Design review of the part built by this model. Coordinates are the model's own, in mm. A direction names the side the tool comes from. Give positions to 0.01 mm unless a question says otherwise; leave off trailing zeros. Order: outer loops, then holes, each group sorted by start corner. A loop starts at its lowest first (then second) coordinate and runs counter-clockwise, first axis right, second up. Notation, with made-up numbers: (80.25, 1.25) -> (131.25, 1.25) arc R11 ccw to (131.25, 10.25) -> close; hole circle Ø4 at (-26.5, -29.5). An arc over 180 degrees is marked (long way). One line per item, written item: value.
from build123d import *

# Parameters (mm, degrees)
SKETCH_1_R          = 40
EXTRUDE_1_DEPTH     = 30
CUT_EXTRUDE_1_DEPTH = 31


with BuildPart() as part:
    # 草图1 → 凸台-拉伸1 (new body)
    with BuildSketch(Plane(origin=(0, 0, 0), x_dir=(0, 0, -1), z_dir=(1, 0, 0))):
        Circle(SKETCH_1_R)
    extrude(amount=EXTRUDE_1_DEPTH)

    # 草图2 → 切除-拉伸1 (cut, through all)
    with BuildSketch(Plane(origin=(0, 0, 0), x_dir=(0, 0, -1), z_dir=(1, 0, 0))):
        with BuildLine():
            Line((2.623542319, -4.321331792), (7.918602352, -9.756071778))
            Line((7.918602352, -9.756071778), (9.351104694, -8.360386627))
            Line((9.351104694, -8.360386627), (4.055722569, -2.925316052))
            ThreePointArc((4.055722569, -2.925316052), (3.501362158, 3.37399969), (-2.781388072, 4.092152751))
            Line((-2.781388072, 4.092152751), (-8.094959692, 9.545892647))
            Line((-8.094959692, 9.545892647), (-9.527462034, 8.150207496))
            Line((-9.527462034, 8.150207496), (-4.214212506, 2.696798189))
            ThreePointArc((-4.214212506, 2.696798189), (-3.661149551, -3.604426065), (2.623542319, -4.321331792))
        make_face()
    extrude(amount=CUT_EXTRUDE_1_DEPTH, mode=Mode.SUBTRACT)


solid = part.part
Item 1: Add section C-C on y = 0. Give the boundary of the cut face in (x, z), plus the area to 3 significant figures.
Returned:
outline: (0, -40) -> (30, -40) -> (30, -4.92) -> (0, -4.92) -> close; (0, 5.08) -> (30, 5.08) -> (30, 40) -> (0, 40) -> close
area: 2,100 mm²
Item 2: Add section D-D on y = -16.5. Give the boundary of the cut face in (x, z).
Returned:
outline: (0, -36.44) -> (30, -36.44) -> (30, 36.44) -> (0, 36.44) -> close
Item 3: Add section B-B on z = 0. Give the boundary of the cut face in (x, y).
Returned:
outline: (0, -40) -> (30, -40) -> (30, -5.11) -> (0, -5.11) -> close; (0, 4.88) -> (30, 4.88) -> (30, 40) -> (0, 40) -> close
Item 4: Machinability: for faces 1 (the flat face through (14.79, 6.78, 5.4)), 2 (the flat face through (0, 1, -8)), which of the approach directions +Z, -Z, +X, -X, +Y, -Y give a long, thin tool a straight path to every point of the face, cutting with its end or side? Answer none if there is none.
Returned:
face 1: +X, -X
face 2: +Z, -Z, -X, +Y, -Y
Item 5: To check wall thickness, follow line 1 along Y through (x, z) = (9.5, -8); line 2 along Z through (x, y) = (22, 3); line 3 along Z through (x, y) = (28, -7.5). State the ranges of each line that lie inside material, in increasing order. Write a range as from..to.
Returned:
line 1: -39.19..-9.68, -6.97..39.19
line 2: -39.89..-3.83, 4.51..39.89
line 3: -39.29..-8.51, -5.72..39.29
Item 6: Clearance check with flat-ended pins moving along their axes: P1, Ø2, axis at x = 5.5, y = 1, coming from the -Z side; P2, Ø1, axis at x = 19, z = -23, coming from the -Y side; P3, Ø3, axis at x = 19.5, y = 7.5, coming from the +Z side; P4, Ø8, axis at x = 4, y = 9.5, coming from the -Z side. State where each tip first meets the part, or that it passes through.
Returned:
P1: z = -40
P2: y = -33.07
P3: z = 39.55
P4: z = -39.62
Item 7: Add section A-A on x = 4. Give the boundary of the cut face in (y, z), plus the area to 3 significant figures.
Returned:
outline: circle Ø80 at (0, 0); hole (-9.76, -7.92) -> (-8.36, -9.35) -> (-2.93, -4.06) arc R5 ccw to (4.09, 2.78) -> (9.55, 8.09) -> (8.15, 9.53) -> (2.7, 4.21) arc R5 ccw to (-4.32, -2.62) -> close
area: 4,920 mm²
Item 8: Draft analysis for pull direction Z (two halves, no side actions). For faces 3 (the flat face through (14.79, -7.001, -5.234)), 4 (the flat face through (30, 1, -8)), 5 (the cylindrical face through (14.79, -39.05, 8.67)), state which applies: pulls with the +Z half, pulls with the -Z half, needs draft (parallel to the pull), parting line crosses it, or undercut.
Returned:
face 3: undercut
face 4: needs draft
face 5: parting line crosses it
